Autodesk Inventor part; units mm, degrees
ref_plane "Work Plane2" through (-26.5401, 7.7836, 6.83) normal (0, 0, -1) x (0, 1, 0)
ref_plane "YZ Plane" through (0, 0, 0) normal (1, 0, 0) x (0, 1, 0)
ref_plane "XZ Plane" through (0, 0, 0) normal (0, 1, 0) x (-1, 0, 0)
ref_plane "Work Plane1" through (0, 0, 0) normal (0, 0, 1) x (1, 0, 0)
sketch "Sketch1" plane through (0, 0, 0) normal (0, 0, 1) x (1, 0, 0)
  arc A0 (80, 65) -> (65, 80) centre (65, 65) ccw
  line L0 (80, 65) -> (80, -65)
  arc A1 (65, -80) -> (80, -65) centre (65, -65) ccw
  line L1 (65, -80) -> (-65, -80)
  arc A2 (-80, -65) -> (-65, -80) centre (-65, -65) ccw
  line L2 (-80, -65) -> (-80, 65)
  arc A3 (-65, 80) -> (-80, 65) centre (-65, 65) ccw
  line L3 (-65, 80) -> (65, 80)
  line L4 (-150, -150) -> (150, -150)
  line L5 (150, -150) -> (150, 150)
  line L6 (150, 150) -> (-150, 150)
  line L7 (-150, 150) -> (-150, -150)
  line L8 (79, -65) -> (79, 65)
  arc A4 (79, 65) -> (65, 79) centre (65, 65) ccw
  line L9 (65, 79) -> (-65, 79)
  arc A5 (-65, 79) -> (-79, 65) centre (-65, 65) ccw
  line L10 (-79, 65) -> (-79, -65)
  arc A6 (-79, -65) -> (-65, -79) centre (-65, -65) ccw
  line L11 (-65, -79) -> (65, -79)
  arc A7 (65, -79) -> (79, -65) centre (65, -65) ccw
  circle A8 centre (-67, -107.5) radius 1.95
  circle A9 centre (67, 107.5) radius 1.95
  circle A10 centre (-67, 107.5) radius 1.95
  circle A11 centre (67, -107.5) radius 1.95
  point P0 (0, 0)
  dimension "d0" = 1
ref_plane "Work Plane3" through (0, 0, 0) normal (0, 0, 1) x (1, 0, 0)
sketch "Sketch2" plane through (0, 0, 0) normal (0, 0, 1) x (1, 0, 0)
  line L0 (79, -65) -> (79, 65)
  arc A0 (79, 65) -> (65, 79) centre (65, 65) ccw
  line L1 (65, 79) -> (-65, 79)
  arc A1 (-65, 79) -> (-79, 65) centre (-65, 65) ccw
  line L2 (-79, 65) -> (-79, -65)
  arc A2 (-79, -65) -> (-65, -79) centre (-65, -65) ccw
  line L3 (-65, -79) -> (65, -79)
  arc A3 (65, -79) -> (79, -65) centre (65, -65) ccw
  line L4 (-79, -125) -> (79, -125)
  line L5 (79, -125) -> (79, 125)
  line L6 (79, 125) -> (-79, 125)
  line L7 (-79, 125) -> (-79, -125)
  line L8 (-79, -125) -> (79, 125) construction
  line L9 (79, -125) -> (-79, 125) construction
  point P0 (0, 0)
  dimension "d3" = 250
extrude "Extrusion2" add sketch "Sketch2" along normal blind 4
ref_plane "Work Plane2" through (-26.5401, 7.7836, 6.83) normal (0, 0, -1) x (0, 1, 0)
sketch "Sketch3" plane through (0, 0, 4) normal (0, 0, 1) x (1, 0, 0)
  arc A0 (-22.3322, 15.5836) -> (-25.0072, 11.4836) centre (-3.6319, 0.4603) ccw
  line L0 (-21.3013, 11.4836) -> (-25.0072, 11.4836)
  arc A1 (-21.3013, 11.4836) -> (-20.1013, 15.0836) centre (-21.3013, 13.4836) ccw
  line L1 (-20.1013, 15.5836) -> (-20.1013, 15.0836)
  line L2 (-22.3322, 15.5836) -> (-20.1013, 15.5836)
  circle A2 centre (-21.3013, 13.4836) radius 0.9
  circle A3 centre (6.0928, 10.7836) radius 1.575
  circle A4 centre (6.0928, 10.7836) radius 0.7
  circle A5 centre (4.2678, -11.3664) radius 1.575
  circle A6 centre (4.2678, -11.3664) radius 0.7
  circle A7 centre (-21.3013, 13.4836) radius 0.9
  circle A8 centre (-21.3013, 13.4836) radius 2
  circle A9 centre (25.4178, -3.2164) radius 0.9
  circle A10 centre (-20.4322, -13.5164) radius 0.9
  circle A11 centre (-20.4322, -13.5164) radius 2
  circle A12 centre (25.4178, -3.2164) radius 2
  point P0 (0, 0)
extrude "Extrusion3" add sketch "Sketch3" along normal up to surface (2.83 mm away) contours A8 A1 | A11 | A12
sketch "Sketch4" plane through (25.4178, -3.2164, 6.83) normal (0, 0, 1) x (1, 0, 0)
  circle A0 centre (0, 0) radius 2
  circle A1 centre (0, 0) radius 0.9
  point P0 (-25.4178, 3.2164)
extrude "Extrusion4" add sketch "Sketch4" along normal up to surface (1.2 mm away)
sketch "Sketch5" plane through (0, 0, 4) normal (0, 0, 1) x (1, 0, 0)
  circle A0 centre (-20.4322, -13.5164) radius 2
  circle A1 centre (-20.4322, -13.5164) radius 0.9
  circle A2 centre (-21.3013, 13.4836) radius 0.9
  circle A3 centre (25.4178, -3.2164) radius 0.9
  point P0 (0, 0)
extrude "Extrusion5" cut sketch "Sketch5" against normal through all contours A1 | A2 | A3
sketch "Sketch6" plane through (0, 0, 4) normal (0, 0, 1) x (1, 0, 0)
  circle A0 centre (76, -85) radius 1.95
  circle A1 centre (26, -85) radius 1.95
  circle A2 centre (26, -35) radius 1.95
  circle A3 centre (76, -35) radius 1.95
  circle A4 centre (76, 35) radius 1.95
  circle A5 centre (26, 35) radius 1.95
  circle A6 centre (76, 85) radius 1.95
  circle A7 centre (26, 85) radius 1.95
  point P0 (0, 0)
extrude "Extrusion6" cut sketch "Sketch6" against normal through all
sketch "Sketch7" plane through (0, 0, 0) normal (0, 0, -1) x (-1, 0, 0)
  circle A0 centre (-76, 85) radius 1.95
  circle A1 centre (-76, 35) radius 1.95
  circle A2 centre (-26, -35) radius 1.95
  circle A3 centre (-76, -85) radius 1.95
  circle A4 centre (-26, -85) radius 1.95
  circle A5 centre (-76, -35) radius 1.95
  circle A6 centre (-26, 35) radius 1.95
  circle A7 centre (-26, 85) radius 1.95
  line L0 (79, -125) -> (-79, -125)
  line L1 (79, 125) -> (79, -125)
  line L2 (-79, 125) -> (79, 125)
  line L3 (-79, -125) -> (-79, 125)
  line L4 (67, -107.5) -> (-67, -107.5)
  line L5 (-67, -107.5) -> (-67, 107.5)
  line L6 (-67, 107.5) -> (67, 107.5)
  line L7 (67, 107.5) -> (67, -107.5)
  line L8 (67, -107.5) -> (-67, 107.5) construction
  line L9 (-67, -107.5) -> (67, 107.5) construction
  point P0 (0, 0)
  dimension "d16" = 134
  dimension "d17" = 215
hole "Hole1" at (-67, 107.5, 0) at (67, 107.5, 0) at (67, -107.5, 0) at (-67, -107.5, 0) direction (0, 0, 1) diameter 3.9 depth 10 tip angle 118
properties part number "01_Zeiss_Axiotech_adapterplate"
Work out the finished part from the listing and answer in its coordinate system (mm). Give positions to 0.01 mm unless a question says otherwise; leave off trailing zeros. Loops run counter-clockwise (first coordinate to the right, second up) from the corner with the lowest first, then second, coordinate; pieces in that order, holes last. Notation, with made-up numbers: (-24.5, -5) -> (32.5, -5) arc R16 ccw to (32.5, 22) -> close; hole circle Ø7 at (-36.5, 9.25). An arc over 180 degrees is marked (long way). Put each result on its own line as item: value. Start each with the question number.
Item 1: Each of these flat-tipped pins is pushed along its axis until it touches: P1, Ø2, axis at x = -19.5, y = -13, coming from the +Z side; P2, Ø3.5, axis at x = 26, y = -35, coming from the +Z side; P3, Ø5, axis at x = 26, y = 85, coming from the +Z side. Where does it stop, or does it pass through?
Item 2: The part is cut by section B-B (x = -40). Give the vertices of the cut face in (y, z).
Item 3: Find the intervals of material crossed by L1, parallel to X at y = -107.5, z = 1.45; L2, parallel to Y at x = 26, z = 1.2; L3, parallel to Z at x = 27.5, y = -16.5, in increasing order. Write a range as [from, to].
Item 4: The part is cut by section A-A (y = 67.5). Give the vertices of the cut face in (x, z), then the cut area to 3 significant figures.
Answers below:
1. P1: z = 6.83
1. P2: through
1. P3: z = 4
2. outline: (-125, 0) -> (125, 0) -> (125, 4) -> (-125, 4) -> close
3. L1: [-79, -68.95], [-65.05, 65.05], [68.95, 79]
3. L2: [-125, -86.95], [-83.05, -36.95], [-33.05, -3.9], [-2.53, 33.05], [36.95, 83.05], [86.95, 125]
3. L3: [0, 4]
4. outline: (-79, 0) -> (79, 0) -> (79, 4) -> (-79, 4) -> close
4. area: 632 mm2
